The drawing under review shows one solid part. Ordinate dimensions are in mm from its lowest x, y, z. Coordinates: 2 decimals unless noted, no trailing zeros. Order: outer loops, then holes, each group sorted by start corner. A loop starts at its lowest first (then second) coordinate and runs counter-clockwise, first axis right, second up.
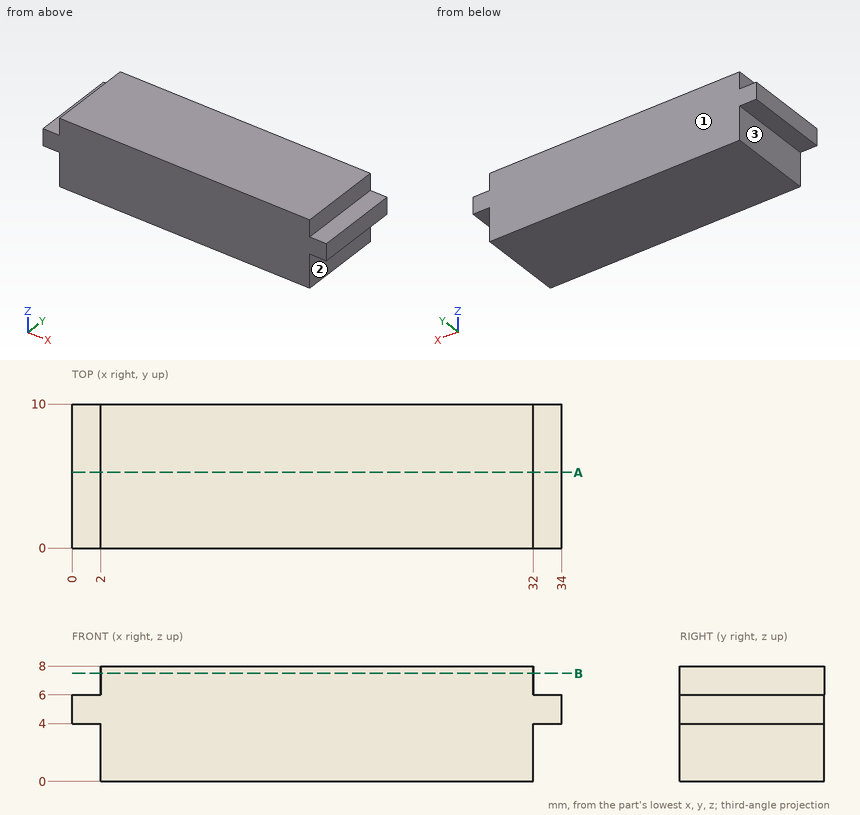
(1) We need section A-A, the plane y = 5.25. Write out the cut boundary in (x, z), and give its area (3 significant figures).
A:
outline: (0, 4) - (2, 4) - (2, 0) - (32, 0) - (32, 4) - (34, 4) - (34, 6) - (32, 6) - (32, 8) - (2, 8) - (2, 6) - (0, 6) - close
area: 248 mm2
(2) Wall thickness on probe 1 along X at (y, z) = (1.75, 1.5): over which ranges is the line inside the solid? List them lowest first.
A:
probe 1: x = 2 to 32
(3) For pin 1 Ø0.6 at (x, y) = (33, 4.5) entering from -Z; pin 2 Ø1.6 at (y, z) = (4.5, 6.5) entering from -X; pin 3 Ø2 at (y, z) = (3, 2.5) entering from +X; pin 4 Ø1.2 at (y, z) = (5, 3) entering from -X, all flat-tipped, find the tip position at first contact; note any pin that passes through.
A:
pin 1: stops at z = 4
pin 2: stops at x = 0
pin 3: stops at x = 32
pin 4: stops at x = 2
(4) Draft analysis for pull direction X (two halves, no side actions). For the marked faces 1, 2 and 3, state which applies: released by +X, released by -X, zero draft, split by the parting line, or undercut.
A:
face 1: zero draft
face 2: released by +X
face 3: released by -X
(5) We need section B-B, the plane z = 7.5. Write out the cut boundary in (x, y), and give its area (3 significant figures).
A:
outline: (2, 0) - (32, 0) - (32, 10) - (2, 10) - close
area: 300 mm2
